```python
from build123d import *

# Parameters (mm, degrees)
F0_W     = 22.4536
F0_H     = 22.4536
F1_DEPTH = 152.4
F2_R     = 7.9375
F3_DEPTH = 22.4546
F4_R     = 5.1562
F5_DEPTH = 22.4546


with BuildPart() as f1:
    # F0 (on Front) → F1 (new body)
    with BuildSketch(Plane.XZ):
        with Locations((27.084826, 25.844949)):
            Rectangle(F0_W, F0_H)
    extrude(amount=F1_DEPTH)

    # F2 (on face) → F3 (cut, through all)
    with BuildSketch(Plane.XY.offset(37.071749)):
        with Locations((27.084826, -76.2)):
            Circle(F2_R)
    extrude(amount=-F3_DEPTH, mode=Mode.SUBTRACT)

    # F4 (on face) → F5 (cut, through all)
    with BuildSketch(Plane.YZ.offset(38.311626)):
        with Locations((-139.7, 25.844949)):
            Circle(F4_R)
        with Locations((-12.7, 25.844949)):
            Circle(F4_R)
    extrude(amount=-F5_DEPTH, mode=Mode.SUBTRACT)


solid = f1.part
```
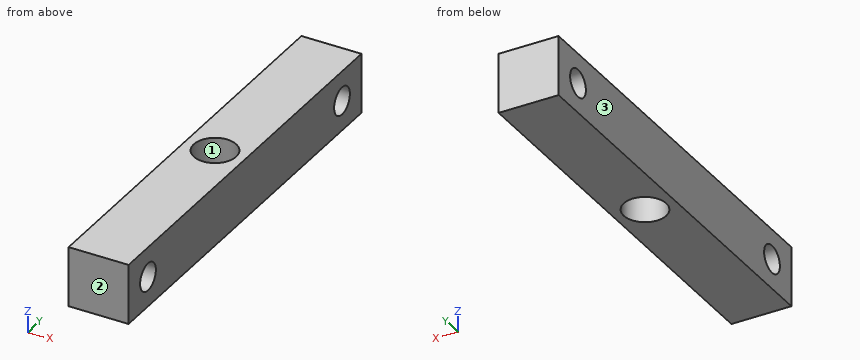
Check sheet for the modelled part. Datum: model origin and axes. Units: mm. Face numbers are marked on the shaded views. Give positions to 0.01 mm unless a question says otherwise; leave off trailing zeros. Order: outer loops, then holes, each group sorted by start corner. A loop starts at its lowest first (then second) coordinate and runs counter-clockwise, first axis right, second up. Notation, with made-up numbers: (24.25, 41.5) -> (80.25, 41.5) arc R32 cw to (80.25, 80.5) -> close; hole circle Ø6 at (40.5, 40.25). An arc over 180 degrees is marked (long way). Return JSON: item names as keys, results as strings.
1. Go/stop test with a flat-tipped pin: P1, Ø9.5, axis at y = -12.7, z = 25.84, coming from the +X side. Record where the tip stops, or that it passes through.
From the geometry:
{"P1": "through"}
2. Cross-section at B-B, the plane z = 24.5. Record the cut outline in (x, y) (1 decimal), plus the area to 3 significant figures.
From the geometry:
{"outline": "(15.9, -152.4) -> (38.3, -152.4) -> (38.3, -144.7) -> (15.9, -144.7) -> close; (15.9, -134.7) -> (38.3, -134.7) -> (38.3, -17.7) -> (15.9, -17.7) -> close; (15.9, -7.7) -> (38.3, -7.7) -> (38.3, 0) -> (15.9, 0) -> close; hole circle Ø15.9 at (27.1, -76.2)", "area": "2,780 mm^2"}
3. Cross-section at D-D, the plane x = 22. Record the cut outline in (y, z), plus the area to 3 significant figures.
From the geometry:
{"outline": "(-152.4, 14.62) -> (-82.29, 14.62) -> (-82.29, 37.07) -> (-152.4, 37.07) -> close; (-70.11, 14.62) -> (0, 14.62) -> (0, 37.07) -> (-70.11, 37.07) -> close; hole circle Ø10.31 at (-139.7, 25.84); hole circle Ø10.31 at (-12.7, 25.84)", "area": "2,980 mm^2"}
4. Mould release check, pull along X, two halves, no side actions. Record for the marked faces 1, 2 and 3: +X half, -X half, draft (parallel to the pull), parting line (faces both ways), or undercut.
From the geometry:
{"face 1": "undercut", "face 2": "draft", "face 3": "-X half"}
5. Cross-section at C-C, the plane y = -139.7. Record the cut outline in (x, z).
From the geometry:
{"outline": "(15.86, 14.62) -> (38.31, 14.62) -> (38.31, 20.69) -> (15.86, 20.69) -> close; (15.86, 31) -> (38.31, 31) -> (38.31, 37.07) -> (15.86, 37.07) -> close"}
6. Material ranges on probe 1 along Y at (x, z) = (17, 26); probe 2 along Z at (x, y) = (33, -12.7); probe 3 along Y at (x, z) = (25.75, 26.75), recorded low to high. Write a range as [from, to].
From the geometry:
{"probe 1": "[-152.4, -144.85], [-134.55, -17.85], [-7.55, 0]", "probe 2": "[14.62, 20.69], [31, 37.07]", "probe 3": "[-152.4, -144.78], [-134.62, -84.02], [-68.38, -17.78], [-7.62, 0]"}
7. Cross-section at A-A, the plane x = 29.5. Record the cut outline in (y, z).
From the geometry:
{"outline": "(-152.4, 14.62) -> (-83.76, 14.62) -> (-83.76, 37.07) -> (-152.4, 37.07) -> close; (-68.64, 14.62) -> (0, 14.62) -> (0, 37.07) -> (-68.64, 37.07) -> close; hole circle Ø10.31 at (-139.7, 25.84); hole circle Ø10.31 at (-12.7, 25.84)"}
